from build123d import *
from OCP.BRepFilletAPI import BRepFilletAPI_MakeChamfer

# Parameters (mm, degrees)
SKETCH1_W           = 4
SKETCH1_H           = 13.20710931
BOSS_EXTRUDE1_DEPTH = 1.5
BOSS_EXTRUDE7_START = 1.5
SKETCH1_10_W        = 1.073289239
SKETCH1_10_H        = 9.306047289
BOSS_EXTRUDE7_DEPTH = 0.75
BOSS_EXTRUDE4_DEPTH = 6.5
SKETCH1_7_R         = 3.125
BOSS_EXTRUDE5_DEPTH = 4
SKETCH1_8_R         = 1.125
BOSS_EXTRUDE6_DEPTH = 5.75
CHAMFER1_SIZE       = 0.25
CHAMFER1_SIZE2      = 0.370640242
CHAMFER2_SIZE       = 0.5
FILLET1_R           = 6
SKETCH2_W           = 13.595412958
SKETCH2_H           = 7
CUT_EXTRUDE1_DEPTH  = 10
FILLET2_R           = 0.5
FILLET3_START       = -1
FILLET3_DEPTH       = 6


with BuildPart() as part:
    # Sketch1 → Boss-Extrude1 (new body)
    with BuildSketch(Plane(origin=(0, 0, 0), x_dir=(1, 0, 0), z_dir=(0, 1, 0))):
        with BuildLine():
            Line((10.25, 11.75), (-10.25, 11.75))
            ThreePointArc((-10.25, 11.75), (-11.310660172, 11.310660172), (-11.75, 10.25))
            Line((-11.75, 10.25), (-11.75, -10.25))
            ThreePointArc((-11.75, -10.25), (-11.310660172, -11.310660172), (-10.25, -11.75))
            Line((-10.25, -11.75), (10.25, -11.75))
            ThreePointArc((10.25, -11.75), (11.310660172, -11.310660172), (11.75, -10.25))
            Line((11.75, -10.25), (11.75, 10.25))
            ThreePointArc((11.75, 10.25), (11.310660172, 11.310660172), (10.25, 11.75))
        make_face()
        with Locations((-9, 0.048761158)):
            Rectangle(SKETCH1_W, SKETCH1_H, mode=Mode.SUBTRACT)
        Polygon((11, -6.554793497), (7, -6.554793497), (7, -3.401386803), (2.793672018, -3.401386803), (2.793672018, 3.417114723), (7, 3.417114723), (7, 6.652315813), (11, 6.652315813), align=None, mode=Mode.SUBTRACT)
    extrude(amount=BOSS_EXTRUDE1_DEPTH)

    # Sketch1<10> → Boss-Extrude7 (add)
    with BuildSketch(Plane(origin=(0, 0, 0), x_dir=(1, 0, 0), z_dir=(0, 1, 0)).offset(BOSS_EXTRUDE7_START)):
        with Locations((-5.639254257, 0.06795853)):
            Rectangle(SKETCH1_10_W, SKETCH1_10_H)
    extrude(amount=BOSS_EXTRUDE7_DEPTH)

    # Sketch1<6> → Boss-Extrude4 (add)
    with BuildSketch(Plane(origin=(0, 0, 0), x_dir=(1, 0, 0), z_dir=(0, 1, 0))):
        with BuildLine():
            Line((10.25, 13.75), (-10.25, 13.75))
            ThreePointArc((-10.25, 13.75), (-11.386617955, 13.560302044), (-12.400027852, 13.011771214))
            ThreePointArc((-12.400027852, 13.011771214), (-12.694859313, 12.694859313), (-13.011771214, 12.400027852))
            ThreePointArc((-13.011771214, 12.400027852), (-13.560302044, 11.386617955), (-13.75, 10.25))
            Line((-13.75, 10.25), (-13.75, -10.25))
            ThreePointArc((-13.75, -10.25), (-13.560302044, -11.386617955), (-13.011771214, -12.400027852))
            ThreePointArc((-13.011771214, -12.400027852), (-12.694859313, -12.694859313), (-12.400027852, -13.011771214))
            ThreePointArc((-12.400027852, -13.011771214), (-11.386617955, -13.560302044), (-10.25, -13.75))
            Line((-10.25, -13.75), (10.25, -13.75))
            ThreePointArc((10.25, -13.75), (11.386617955, -13.560302044), (12.400027852, -13.011771214))
            ThreePointArc((12.400027852, -13.011771214), (12.694859313, -12.694859313), (13.011771214, -12.400027852))
            ThreePointArc((13.011771214, -12.400027852), (13.560302044, -11.386617955), (13.75, -10.25))
            Line((13.75, -10.25), (13.75, 10.25))
            ThreePointArc((13.75, 10.25), (13.560302044, 11.386617955), (13.011771214, 12.400027852))
            ThreePointArc((13.011771214, 12.400027852), (12.694859313, 12.694859313), (12.400027852, 13.011771214))
            ThreePointArc((12.400027852, 13.011771214), (11.386617955, 13.560302044), (10.25, 13.75))
        make_face()
        with BuildLine():
            ThreePointArc((-11.75, 10.25), (-11.310660172, 11.310660172), (-10.25, 11.75))
            Line((-10.25, 11.75), (10.25, 11.75))
            ThreePointArc((10.25, 11.75), (11.310660172, 11.310660172), (11.75, 10.25))
            Line((11.75, 10.25), (11.75, -10.25))
            ThreePointArc((11.75, -10.25), (11.310660172, -11.310660172), (10.25, -11.75))
            Line((10.25, -11.75), (-10.25, -11.75))
            ThreePointArc((-10.25, -11.75), (-11.310660172, -11.310660172), (-11.75, -10.25))
            Line((-11.75, -10.25), (-11.75, 10.25))
        make_face(mode=Mode.SUBTRACT)
    extrude(amount=BOSS_EXTRUDE4_DEPTH)

    # Sketch1<7> → Boss-Extrude5 (add)
    with BuildSketch(Plane(origin=(0, 0, 0), x_dir=(1, 0, 0), z_dir=(0, 1, 0))):
        with BuildLine():
            ThreePointArc((19.817252096, -11.673753439), (23, 0), (19.817252096, 11.673753439))
            ThreePointArc((19.817252096, 11.673753439), (21.180140687, 21.180140687), (11.673753439, 19.817252096))
            ThreePointArc((11.673753439, 19.817252096), (0, 23), (-11.673753439, 19.817252096))
            ThreePointArc((-11.673753439, 19.817252096), (-21.180140687, 21.180140687), (-19.817252096, 11.673753439))
            ThreePointArc((-19.817252096, 11.673753439), (-23, 0), (-19.817252096, -11.673753439))
            ThreePointArc((-19.817252096, -11.673753439), (-21.180140687, -21.180140687), (-11.673753439, -19.817252096))
            ThreePointArc((-11.673753439, -19.817252096), (0, -23), (11.673753439, -19.817252096))
            ThreePointArc((11.673753439, -19.817252096), (21.180140687, -21.180140687), (19.817252096, -11.673753439))
        make_face()
        with BuildLine():
            Line((-10.25, 13.75), (10.25, 13.75))
            ThreePointArc((10.25, 13.75), (12.724873734, 12.724873734), (13.75, 10.25))
            Line((13.75, 10.25), (13.75, -10.25))
            ThreePointArc((13.75, -10.25), (12.724873734, -12.724873734), (10.25, -13.75))
            Line((10.25, -13.75), (-10.25, -13.75))
            ThreePointArc((-10.25, -13.75), (-12.724873734, -12.724873734), (-13.75, -10.25))
            Line((-13.75, -10.25), (-13.75, 10.25))
            ThreePointArc((-13.75, 10.25), (-12.724873734, 12.724873734), (-10.25, 13.75))
        make_face(mode=Mode.SUBTRACT)
        with Locations(Location((-16.9375, -16.9375, 0), (0, 0, 270))):
            Circle(SKETCH1_7_R, mode=Mode.SUBTRACT)
        with Locations(Location((-16.9375, 16.9375, 0), (0, 0, 270))):
            Circle(SKETCH1_7_R, mode=Mode.SUBTRACT)
        with Locations(Location((16.9375, 16.9375, 0), (0, 0, 270))):
            Circle(SKETCH1_7_R, mode=Mode.SUBTRACT)
        with Locations(Location((16.9375, -16.9375, 0), (0, 0, 270))):
            Circle(SKETCH1_7_R, mode=Mode.SUBTRACT)
    extrude(amount=BOSS_EXTRUDE5_DEPTH)

    # Sketch1<8> → Boss-Extrude6 (add)
    with BuildSketch(Plane(origin=(0, 0, 0), x_dir=(1, 0, 0), z_dir=(0, 1, 0))):
        with Locations(Location((-8.65, 8.65, 0), (0, 0, 270))):
            Circle(SKETCH1_8_R)
        with Locations(Location((8.65, 8.65, 0), (0, 0, 270))):
            Circle(SKETCH1_8_R)
        with Locations(Location((-8.65, -8.65, 0), (0, 0, 270))):
            Circle(SKETCH1_8_R)
        with Locations(Location((8.65, -8.65, 0), (0, 0, 270))):
            Circle(SKETCH1_8_R)
    extrude(amount=BOSS_EXTRUDE6_DEPTH)

    # Chamfer1: one chamfer whose edges measure the first distance from different faces: ONE call of the kernel's chamfer builder (chamfer() names one face for all edges)
    chamfer1_edges_1 = [part.edges().sort_by_distance(p)[0] for p in [
        (-8.65, 5.75, -9.775),
    ]]
    chamfer1_side_1 = [part.faces().sort_by_distance(p)[0] for p in [
        (-8.65, 3.625, -9.775),
    ]]
    chamfer1_edges_2 = [part.edges().sort_by_distance(p)[0] for p in [
        (8.65, 5.75, -9.775),
    ]]
    chamfer1_side_2 = [part.faces().sort_by_distance(p)[0] for p in [
        (8.65, 3.625, -9.775),
    ]]
    chamfer1_edges_3 = [part.edges().sort_by_distance(p)[0] for p in [
        (8.65, 5.75, 7.525),
    ]]
    chamfer1_side_3 = [part.faces().sort_by_distance(p)[0] for p in [
        (8.65, 3.625, 7.525),
    ]]
    chamfer1_edges_4 = [part.edges().sort_by_distance(p)[0] for p in [
        (-8.65, 5.75, 7.525),
    ]]
    chamfer1_side_4 = [part.faces().sort_by_distance(p)[0] for p in [
        (-8.65, 3.625, 7.525),
    ]]
    chamfer1 = BRepFilletAPI_MakeChamfer(part.part.solid().wrapped)
    for e in chamfer1_edges_1:
        chamfer1.Add(CHAMFER1_SIZE, CHAMFER1_SIZE2, e.wrapped, chamfer1_side_1[0].wrapped)  # the first distance lies on this face
    for e in chamfer1_edges_2:
        chamfer1.Add(CHAMFER1_SIZE, CHAMFER1_SIZE2, e.wrapped, chamfer1_side_2[0].wrapped)  # the first distance lies on this face
    for e in chamfer1_edges_3:
        chamfer1.Add(CHAMFER1_SIZE, CHAMFER1_SIZE2, e.wrapped, chamfer1_side_3[0].wrapped)  # the first distance lies on this face
    for e in chamfer1_edges_4:
        chamfer1.Add(CHAMFER1_SIZE, CHAMFER1_SIZE2, e.wrapped, chamfer1_side_4[0].wrapped)  # the first distance lies on this face
    add(Compound.cast(chamfer1.Shape()), mode=Mode.REPLACE)

    # Chamfer2
    chamfer2_edges = [part.edges().sort_by_distance(p)[0] for p in [
        (16.9375, 4, 13.8125),
        (-16.9375, 0, 13.8125),
        (16.9375, 0, -20.0625),
        (-16.9375, 4, -20.0625),
        (16.9375, 4, -20.0625),
        (-16.9375, 4, 13.8125),
        (-16.9375, 0, -20.0625),
        (16.9375, 0, 13.8125),
    ]]
    chamfer(chamfer2_edges, length=CHAMFER2_SIZE)

    # Fillet1
    fillet1_edges = [part.edges().sort_by_distance(p)[0] for p in [
        (11.673753439, 2, -19.817252096),
        (-11.673753439, 2, -19.817252096),
        (-19.817252096, 2, -11.673753439),
        (-19.817252096, 2, 11.673753439),
        (-11.673753439, 2, 19.817252096),
        (11.673753439, 2, 19.817252096),
        (19.817252096, 2, 11.673753439),
        (19.817252096, 2, -11.673753439),
    ]]
    fillet(fillet1_edges, radius=FILLET1_R)

    # Sketch2 → Cut-Extrude1 (cut)
    with BuildSketch(Plane(origin=(0, 4, 0), x_dir=(1, 0, 0), z_dir=(0, 1, 0))):
        with Locations((22.11761689, -5.52795482)):
            Rectangle(SKETCH2_W, SKETCH2_H)
    extrude(amount=-CUT_EXTRUDE1_DEPTH, mode=Mode.SUBTRACT)

    # Fillet2
    fillet2_edges = [part.edges().sort_by_distance(p)[0] for p in [
        (15.319910411, 0, 5.52795482),
        (15.319910411, 2, 9.02795482),
        (19.115165802, 0, 2.02795482),
        (15.319910411, 2, 2.02795482),
        (18.270000077, 0, 9.02795482),
        (19.115165802, 4, 2.02795482),
        (15.319910411, 4, 5.52795482),
        (18.270000077, 4, 9.02795482),
    ]]
    fillet(fillet2_edges, radius=FILLET2_R)

    # Fillet3: read off the stored shape, not the designer's step
    # Fillet3 outline → Fillet3 (cut)
    with BuildSketch(Plane(origin=(0, 0, 0), x_dir=(1, 0, 0), z_dir=(0, 1, 0)).offset(FILLET3_START)):
        with BuildLine():
            ThreePointArc((22.910420735, -2.027959995), (22.947600473, -1.551654765), (22.974878951, -1.074680039))
            ThreePointArc((22.974878951, -1.074680039), (22.666360474, -1.751392868), (21.975971171, -2.02795482))
            Line((21.975971171, -2.02795482), (22.910420735, -2.027959995))
        make_face()
        with BuildLine():
            ThreePointArc((20.058455778, -9.02795482), (20.787477444, -9.343464199), (21.056472764, -10.090899999))
            ThreePointArc((21.056472764, -10.090899999), (21.114417887, -9.555751044), (21.220091225, -9.027948821))
            Line((21.220091225, -9.027948821), (20.058455778, -9.02795482))
        make_face()
    extrude(amount=FILLET3_DEPTH, mode=Mode.SUBTRACT)


solid = part.part
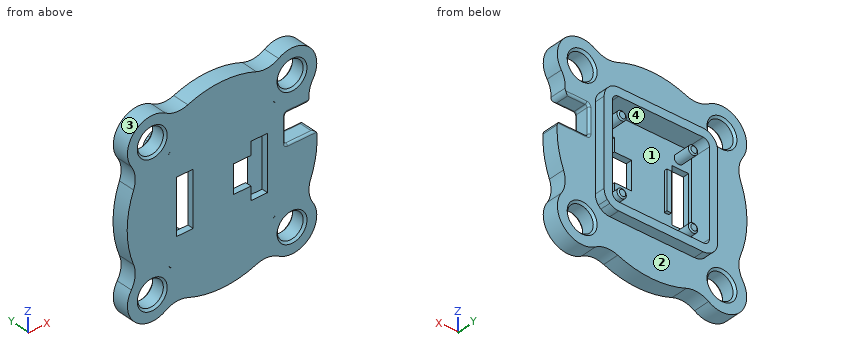
Input: part model. Units: mm. Frame: model coordinates. Face numbers are marked on the shaded views. A direction names the side the tool comes from. Give positions to 0.01 mm unless a question says otherwise; leave off trailing zeros. Write each loop counter-clockwise with the first axis right and the second up, starting at its lowest first coordinate (ties: lowest second). Pieces come first, ordered by that corner, then holes.
Q1. Material intervals for probe 1 along X at (y, z) = (0.5, -6.5); probe 2 along Z at (x, y) = (1, 6), sorted ascending.
Q2. First-contact query: P1, Ø0.8, axis at x = -8.5, y = 0.5, coming from the +Z side; P2, Ø10, axis at x = 14, z = -11, coming from the +Y side; P3, Ø1.7, axis at x = 8.5, z = 8.5, coming from the +Y side; P4, Ø10, axis at x = 16.94, z = -16.94, coming from the +Y side. Flat tips, straight axial feed; report the tip coordinate or a pass-through.
Q3. Section D-D, the plane x = -16. State how many separate pieces and enclosed holes the cut face has, plus the area to 3 significant figures.
Q4. Section A-A, the plane z = -0.5. Output: boundary loops of the cut face in (x, y), plus the area to 3 significant figures.
Q5. Pull-direction query (X, two-part tool) for the marked faces 1 and 2; classes: pulls with the +X half, pulls with the -X half, needs draft (parallel to the pull), parting line crosses it, or undercut.
Q6. Set-up query: the marked faces 3 and 4. Return all of +Z, -Z, +X, -X, +Y, -Y with unobstructed straight access to the full face (end or side cutting, diameter ignored); none if empty.
Q7. Section B-B, the plane x = -4. Output: boundary loops of the cut face in (y, z), plus the area to 3 significant figures.
Q8. Section C-C, the plane z = -6. Output: boundary loops of the cut face in (x, y), plus the area to 3 significant figures.
Filled in:
1. probe 1: x = -22.06 to -11, -7 to 7, 11 to 22.06
1. probe 2: z = -13.75 to -11.75, 11.75 to 13.75
2. P1: stops at z = 21.53
2. P2: stops at y = 6.5
2. P3: stops at y = 5.75
2. P4: stops at y = 4
3. separate pieces: 3
3. enclosed holes: 0
3. area: 134 mm2
4. outline: (-22.99, 0) - (-11, 0) - (-11, 1.5) - (-11.75, 1.5) - (-11.75, 6.5) - (-13.75, 6.5) - (-13.75, 4) - (-22.99, 4) - close; (-7, 0) - (2.79, 0) - (2.79, 1.5) - (-5.1, 1.5) - (-5.1, 2.25) - (-6.18, 2.25) - (-6.18, 1.5) - (-7, 1.5) - close; (11, 0) - (22.99, 0) - (22.99, 4) - (13.75, 4) - (13.75, 6.5) - (11.75, 6.5) - (11.75, 1.5) - (11, 1.5) - close
4. area: 118 mm2
5. face 1: undercut
5. face 2: needs draft
6. face 3: +Y, -Y
6. face 4: +Y
7. outline: (0, -22.65) - (4, -22.65) - (4, -13.75) - (6.5, -13.75) - (6.5, -11.75) - (1.5, -11.75) - (1.5, 11.75) - (6.5, 11.75) - (6.5, 13.75) - (4, 13.75) - (4, 22.65) - (0, 22.65) - close
7. area: 132 mm2
8. outline: (-22.2, 0) - (-11, 0) - (-11, 1.5) - (-11.75, 1.5) - (-11.75, 6.5) - (-13.75, 6.5) - (-13.75, 4) - (-22.2, 4) - close; (-7, 0) - (7, 0) - (7, 1.5) - (-7, 1.5) - close; (11, 0) - (22.2, 0) - (22.2, 4) - (13.75, 4) - (13.75, 6.5) - (11.75, 6.5) - (11.75, 1.5) - (11, 1.5) - close
8. area: 117 mm2
